Build history of the part. All positions in model axes, mm. Face numbers are marked on the shaded views. Round coordinates to 2 decimals unless told otherwise and drop trailing zeros. Write each loop counter-clockwise with the first axis right and the second up, starting at its lowest first coordinate (ties: lowest second). Pieces come first, ordered by that corner, then holes. Notation, with made-up numbers: M 73.5,53.5 L 93.5,53.5 A12 ccw 93.5,58.5 Z; hole C -15,48 d4. An arc over 180 degrees is marked long. Use a Markdown table: item, result.
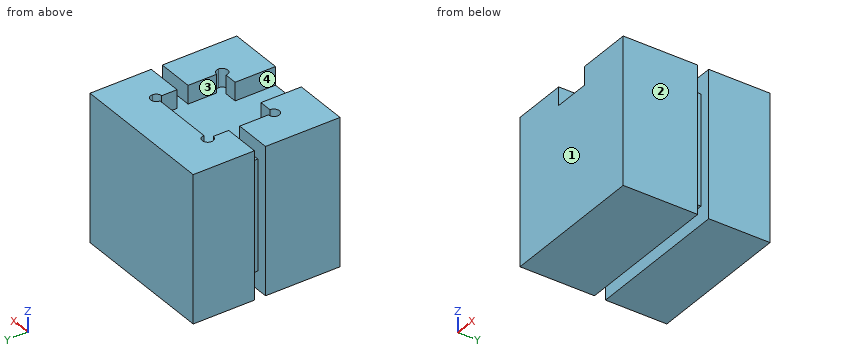
from build123d import *

# Parameters (mm, degrees)
F0_W     = 40
F0_H     = 40
F1_DEPTH = 40
F2_W     = 10
F2_H     = 11
F3_DEPTH = 5
F4_W     = 3
F4_H     = 3
F5_DEPTH = 40.001
F6_W     = 3
F6_H     = 5
F7_DEPTH = 40.001


with BuildPart() as f1:
    # F0 (on Top) → F1 (new body)
    with BuildSketch(Plane.XY):
        Rectangle(F0_W, F0_H)
    extrude(amount=F1_DEPTH)

    # F2 (on face) → F3 (cut)
    with BuildSketch(Plane.XY.offset(40)):
        with BuildLine():
            ThreePointArc((-10, 7.5), (-8.9393398282, 7.9393398282), (-8.5, 9))
            Line((-8.5, 9), (-10, 9))
            Line((-10, 9), (-10, 7.5))
        make_face()
        with BuildLine():
            Line((-10, 9), (-8.5, 9))
            ThreePointArc((-8.5, 9), (-11.0606601718, 10.0606601718), (-10, 7.5))
            Line((-10, 7.5), (-10, 9))
        make_face()
        with BuildLine():
            Line((8.5, 9), (-8.5, 9))
            ThreePointArc((-8.5, 9), (-8.9393398282, 7.9393398282), (-10, 7.5))
            Line((-10, 7.5), (-10, -7.5))
            ThreePointArc((-10, -7.5), (-8.9393398282, -7.9393398282), (-8.5, -9))
            Line((-8.5, -9), (-5, -9))
            Line((-5, -9), (5, -9))
            Line((5, -9), (8.5, -9))
            ThreePointArc((8.5, -9), (8.9393398282, -7.9393398282), (10, -7.5))
            Line((10, -7.5), (10, 7.5))
            ThreePointArc((10, 7.5), (8.9393398282, 7.9393398282), (8.5, 9))
        make_face()
        with BuildLine():
            ThreePointArc((11.5, 9), (10, 10.5), (8.5, 9))
            Line((8.5, 9), (10, 9))
            Line((10, 9), (10, 7.5))
            ThreePointArc((10, 7.5), (11.0606601718, 7.9393398282), (11.5, 9))
        make_face()
        with BuildLine():
            Line((10, 9), (8.5, 9))
            ThreePointArc((8.5, 9), (8.9393398282, 7.9393398282), (10, 7.5))
            Line((10, 7.5), (10, 9))
        make_face()
        with BuildLine():
            ThreePointArc((-8.5, -9), (-8.9393398282, -7.9393398282), (-10, -7.5))
            Line((-10, -7.5), (-10, -9))
            Line((-10, -9), (-8.5, -9))
        make_face()
        with BuildLine():
            Line((-10, -9), (-10, -7.5))
            ThreePointArc((-10, -7.5), (-11.0606601718, -10.0606601718), (-8.5, -9))
            Line((-8.5, -9), (-10, -9))
        make_face()
        with BuildLine():
            ThreePointArc((11.5, -9), (11.0606601718, -7.9393398282), (10, -7.5))
            Line((10, -7.5), (10, -9))
            Line((10, -9), (8.5, -9))
            ThreePointArc((8.5, -9), (10, -10.5), (11.5, -9))
        make_face()
        with BuildLine():
            Line((10, -9), (10, -7.5))
            ThreePointArc((10, -7.5), (8.9393398282, -7.9393398282), (8.5, -9))
            Line((8.5, -9), (10, -9))
        make_face()
        with Locations((0, -14.5)):
            Rectangle(F2_W, F2_H)
    extrude(amount=-F3_DEPTH, mode=Mode.SUBTRACT)

    # F4 (on face) → F5 (cut, through all)
    with BuildSketch(Plane.XY.offset(40)):
        with Locations((-18.5, 1.8)):
            Rectangle(F4_W, F4_H)
        with Locations((18.5, 1.8)):
            Rectangle(F4_W, F4_H)
    extrude(amount=-F5_DEPTH, mode=Mode.SUBTRACT)

    # F6 (on face) → F7 (cut, through all)
    with BuildSketch(Plane(origin=(-20, 0, 0), x_dir=(0, -1, 0), z_dir=(-1, 0, 0))):
        with Locations((-1.8, 37.5)):
            Rectangle(F6_W, F6_H)
        with Locations((-1.8, 2.5)):
            Rectangle(F6_W, F6_H)
    extrude(amount=-F7_DEPTH, mode=Mode.SUBTRACT)


solid = f1.part
Q1. Cut at B-B on x = 6.5. Give the cut face in (y, z).
Response values:
| item | result |
|---|---|
| outline | M -20,0 L 0.3,0 L 0.3,5 L 3.3,5 L 3.3,0 L 20,0 L 20,40 L 9,40 L 9,35 L -9,35 L -9,40 L -20,40 Z |
Q2. Cut at A-A on x = -13.5. Give the cut face in (y, z).
Response values:
| item | result |
|---|---|
| outline | M -20,0 L 0.3,0 L 0.3,5 L 3.3,5 L 3.3,0 L 20,0 L 20,40 L 3.3,40 L 3.3,35 L 0.3,35 L 0.3,40 L -20,40 Z |
Q3. Drill centre lines: L1, parallel to Z at x = 0.5, y = 3; L2, parallel to Z at x = 8.5, y = -7; L3, parallel to X at y = 0.5, z = 9. Where is each one in solid material? Low to high.
Response values:
| item | result |
|---|---|
| L1 | z = 5 to 35 |
| L2 | z = 0 to 35 |
| L3 | x = -17 to 17 |
Q4. Cut at C-C on x = -0.5. Give the cut face in (y, z).
Response values:
| item | result |
|---|---|
| outline | M -20,0 L 0.3,0 L 0.3,5 L 3.3,5 L 3.3,0 L 20,0 L 20,40 L 9,40 L 9,35 L -20,35 Z |
Q5. Drop flat-ended pins along their axis: P1, Ø1.8, axis at x = -10, y = 9, coming from the +Z side; P2, Ø1.5, axis at y = 2.5, z = 25.5, coming from the -X side. Give the stop position or say it passes through.
Response values:
| item | result |
|---|---|
| P1 | stops at z = 35 |
| P2 | stops at x = -17 |
Q6. Two-plate mould, pull along X, no slides. Class the marked faces 1, 2, 3 and 4: +X half, -X half, draft (parallel to the pull), parting line (faces both ways), or undercut.
Response values:
| item | result |
|---|---|
| face 1 | draft |
| face 2 | +X half |
| face 3 | undercut |
| face 4 | undercut |
